Here's how the part is built. I have some questions about the finished solid (model axes, mm). A direction names the side the tool comes from. Give positions to 0.01 mm unless a question says otherwise; leave off trailing zeros. Write each loop counter-clockwise with the first axis right and the second up, starting at its lowest first coordinate (ties: lowest second). Pieces come first, ordered by that corner, then holes. Notation, with made-up numbers: (-29.75, 24.25) - (5.25, 24.25) arc R17 cw to (5.25, 33.25) - close; hole circle Ø8 at (24, 57). An arc over 180 degrees is marked (long way). One line per item, written item: value. Start each with the question number.
1) We'd pull the mould along Z, two halves only. Please class faces 6 (the flat face through (0, -22, 0)), 7 (the flat face through (-17, -25, 5)), 8 (the cylindrical face through (-24.976, -0.35, 1.099)): +Z half, -Z half, draft (parallel to the pull), parting line (faces both ways), or undercut.
2) I'm going to push flat-ended pins straight in: P1, Ø21, axis at x = 0, z = 0, coming from the -Y side; P2, Ø4, axis at x = -11, y = 9.5, coming from the +Z side; P3, Ø6, axis at y = 12.5, z = 6.5, coming from the -X side. Where does each tip first touch, or does it pass through?
3) Imagine slicing it at B-B on x = -7.5. Write out the boundary of the cut face in (y, z), plus the area to 3 significant figures.
4) Please list where these lines run through material, in increasing order: L1, parallel to Z at x = 0, y = 23.55; L2, parallel to Y at x = 1, z = 16; L3, parallel to Y at x = 30.5, z = 7 (3 decimals). Write a range as [from, to].
5) On a 3-axis mill with a long thin cutter (end or side, diameter ignored), from which of +Z, -Z, +X, -X, +Y, -Y can I reach the whole of each face in a straight line? I mean faces 1 (the cylindrical face through (30.36, -4.336, 19.524)), 2 (the cylindrical face through (-13.887, -23.521, -10.648)), 3 (the flat face through (-17, 25, 5)), 4 (the flat face through (0, 22, 0)), 5 (the flat face through (43, 0, 0)). Say none if no direction works.
6) Imagine slicing it at C-C on x = 28.5. Write out the boundary of the cut face in (y, z), plus the area to 3 significant figures.
7) Imagine slicing it at A-A on x = 0. Write out the boundary of the cut face in (y, z).
Autodesk Fusion 360 part; units mm, degrees
sketch "Sketch1" plane through (0, 0, 0) normal (0, 1, 0) x (1, 0, 0)
  circle A0 centre (0, 0) radius 25
  dimension "d1" = 50
extrude "Extrude2" add sketch "Sketch1" along normal mid plane 50
sketch "Sketch2" plane through (0, -25, 0) normal (0, -1, 0) x (1, 0, 0)
  circle A0 centre (0, 0) radius 25
  circle A1 centre (0, 0) radius 17.5
  dimension "d6" = 35
extrude "Extrude3" cut sketch "Sketch2" against normal blind 3 contours A1
mirror "Mirror1" about plane through (0, 0, 0) normal (0, 1, 0) of "Extrude3"
sketch "Sketch3" plane through (0, 0, 0) normal (1, 0, 0) x (0, 1, 0)
  circle A0 centre (0, 0) radius 20
  dimension "d11" = 40
extrude "Extrude4" add sketch "Sketch3" along normal blind 40
sketch "Sketch4" plane through (40, 0, 0) normal (1, 0, 0) x (0, 1, 0)
  circle A0 centre (0, 0) radius 20
  circle A1 centre (0, 0) radius 17.5
  dimension "d14" = 35
extrude "Extrude5" add sketch "Sketch4" along normal blind 3 contours A1
fillet "Fillet1" radius 2 1 edges at (15, 0, 20)
Numbers:
1. face 6: undercut
1. face 7: draft
1. face 8: parting line
2. P1: y = -22
2. P2: z = 23.32
2. P3: x = -24.75
3. outline: (-25, -23.85) - (25, -23.85) - (25, -15.81) - (22, -15.81) - (22, 15.81) - (25, 15.81) - (25, 23.85) - (-25, 23.85) - (-25, 15.81) - (-22, 15.81) - (-22, -15.81) - (-25, -15.81) - close
3. area: 2,200 mm^2
4. L1: [-25, -17.5], [17.5, 25]
4. L2: [-22, 22]
4. L3: [-18.735, 18.735]
5. face 1: +X
5. face 2: -Y
5. face 3: +Z, -Z, +X, -X, +Y
5. face 4: +Y
5. face 5: +Z, -Z, +X, +Y, -Y
6. outline: circle Ø40 at (0, 0)
6. area: 1,260 mm^2
7. outline: (-25, -25) - (25, -25) - (25, -17.5) - (22, -17.5) - (22, 17.5) - (25, 17.5) - (25, 25) - (-25, 25) - (-25, 17.5) - (-22, 17.5) - (-22, -17.5) - (-25, -17.5) - close
